For this review, take the finished solid that the model builds, in its own axes (mm). A direction names the side the tool comes from. Round coordinates to 2 decimals unless told otherwise and drop trailing zeros. Loops run counter-clockwise (first coordinate to the right, second up) from the corner with the lowest first, then second, coordinate; pieces in that order, holes last.
1) Tool access review of faces 1 (the flat face through (-3, -1, -4)), 2 (the flat face through (-0.85, -0.5, -6.4)): name each direction out of +Z, -Z, +X, -X, +Y, -Y from which nothing blocks a thin tool from reaching the whole face with its end or side.
2) Take a section at B-B (x = 0). State the section outline as (y, z) points, then the cut area to 3 significant figures.
3) Take a section at D-D (x = 1.75). Give the number of separate pieces and of enclosed holes in the cut face, then the cut area to 4 significant figures.
4) Insertion check: pin 1 (1.5 mm diameter, centred on x = 1.5, z = 2.5, fed in from +Y). The pin has a flat end and moves straight along its axis. Give the tip position at first contact, or say it passes through.
5) Take a section at C-C (z = -3). State the section outline as (x, y) points.
6) Wall thickness on L1, parallel to Z at x = -2, y = -0.25; L2, parallel to X at y = -0.4, z = 0; L3, parallel to Z at x = -2.5, y = -0.6: over which ranges is each line inside the solid? List them lowest first.
7) Mouldability with a two-part tool opening along Z and no side actions: class faces 3 (the flat face through (-3, 0, -4)), 4 (the cylindrical face through (-2.3, -0.493, -6.605)), 5 (the cylindrical face through (-0.199, -0.493, 4.796)), 6 (the cylindrical face through (0.173, -0.493, 6.598)) as pulls with the +Z half, pulls with the -Z half, needs draft (parallel to the pull), parting line crosses it, or undercut.
8) Take a section at A-A (z = 0). State the section outline as (x, y) points.
```python
from build123d import *

# Parameters (mm, degrees)
F0_R        = 0.75
F1_DEPTH    = 1
F2_T1_DEPTH = 1
F3_R        = 5


# Not quite as in the source:
# - a fillet or chamfer that OpenCascade refuses, or shapes differently, is made with other operations: its cross-section is extruded or revolved along the edge and cut away or added


with BuildPart() as f1:
    # F0 (on Front) → F1 (new body)
    with BuildSketch(Plane.XZ):
        with BuildLine():
            ThreePointArc((-0.85, -4.7241401334), (0, 4.8), (0.85, -4.7241401334))
            Line((0.85, -4.7241401334), (0.85, -8.0241401334))
            ThreePointArc((0.85, -8.0241401334), (3.2306637909, -7.3940608836), (5.3104097906, -6.0752672975))
            Line((5.3104097906, -6.0752672975), (4.5, -4.3373378932))
            ThreePointArc((4.5, -4.3373378932), (0, 6.6), (-4.5, -4.3373378932))
            Line((-4.5, -4.3373378932), (-5.3104097906, -6.0752672975))
            ThreePointArc((-5.3104097906, -6.0752672975), (-3.2306637909, -7.3940608836), (-0.85, -8.0241401334))
            Line((-0.85, -8.0241401334), (-0.85, -4.7241401334))
        make_face()
        with Locations((-2.1376258958, -5.8730788799)):
            Circle(F0_R, mode=Mode.SUBTRACT)
        with Locations((2.1376258958, -5.8730788799)):
            Circle(F0_R, mode=Mode.SUBTRACT)
    extrude(amount=F1_DEPTH)

    # F2: fillet of radius 10 on 2 edges, made by hand

    # F2_s2 → F2_t1 (join)
    with BuildSketch(Plane.XZ):
        with BuildLine():
            ThreePointArc((-5.9685154732, -2.0889852458), (-5.4360464656, -4.0485437672), (-5.3104097906, -6.0752672975))
            Line((-5.3104097906, -6.0752672975), (-4.5, -4.3373378932))
            ThreePointArc((-4.5, -4.3373378932), (-5.3536180719, -3.2911219818), (-5.9685154732, -2.0889852458))
        make_face()
        with BuildLine():
            ThreePointArc((5.3104097906, -6.0752672975), (5.4360464656, -4.0485437672), (5.9685154732, -2.0889852458))
            ThreePointArc((5.9685154732, -2.0889852458), (5.3536180719, -3.2911219818), (4.5, -4.3373378932))
            Line((4.5, -4.3373378932), (5.3104097906, -6.0752672975))
        make_face()
    extrude(amount=F2_T1_DEPTH)

    # F3
    f3_edges = [f1.edges().sort_by_distance(p)[0] for p in [
        (-5.31041, -0.5, -6.075267),
        (5.31041, -0.5, -6.075267),
    ]]
    fillet(f3_edges, radius=F3_R)


solid = f1.part
```
Response:
1. face 1: +Z, -Z, +X, -X, -Y
1. face 2: -Z, +Y, -Y
2. outline: (-1, 4.8) - (0, 4.8) - (0, 6.6) - (-1, 6.6) - close
2. area: 1.80 mm2
3. separate pieces: 3
3. enclosed holes: 0
3. area: 4.005 mm2
4. pin 1: passes through
5. outline: (-5.67, -1) - (-3.75, -1) - (-3.75, 0) - (-5.67, 0) - close; (3.75, -1) - (5.67, -1) - (5.67, 0) - (3.75, 0) - close
6. L1: z = -7.8 to -6.61, -5.14 to -4.36, 4.36 to 6.28
6. L2: x = -6.39 to -4.8, 4.8 to 6.39
6. L3: z = -7.62 to -6.53, -5.22 to -4.1, 4.1 to 6.09
7. face 3: needs draft
7. face 4: undercut
7. face 5: undercut
7. face 6: parting line crosses it
8. outline: (-6.39, -1) - (-4.8, -1) - (-4.8, 0) - (-6.39, 0) - close; (4.8, -1) - (6.39, -1) - (6.39, 0) - (4.8, 0) - close
